Autodesk Inventor part; units mm, degrees
ref_plane "YZ Plane" through (0, 0, 0) normal (1, 0, 0) x (0, 1, 0)
ref_plane "XZ Plane" through (0, 0, 0) normal (0, 1, 0) x (-1, 0, 0)
ref_plane "XY Plane" through (0, 0, 0) normal (0, 0, 1) x (1, 0, 0)
sketch "Sketch2" plane through (0, 0, 0) normal (0, 1, 0) x (-1, 0, 0)
  line L0 (0, 0) -> (100, 0)
  line L1 (100, 0) -> (100, -100)
  line L2 (100, -100) -> (0, -100)
  line L3 (0, -100) -> (0, 0)
  dimension "d2" = 100
  dimension "d3" = 100
extrude "Extrusion2" add sketch "Sketch2" along normal blind 3
sketch "Sketch3" plane through (0, 0, 0) normal (1, 0, 0) x (0, 0, -1)
  line L0 (0, 0) -> (100, 0)
  line L1 (100, 0) -> (100, 113)
  line L2 (100, 113) -> (0, 113)
  line L3 (0, 113) -> (0, 0)
  dimension "d6" = 100
  dimension "d7" = 113
extrude "Extrusion3" add sketch "Sketch3" along normal blind 3
sketch "Sketch4" plane through (0, 3, 0) normal (0, 0, 1) x (1, 0, 0)
  line L0 (3, -3) -> (-100, -3)
  line L1 (3, -3) -> (-100, -3)
  line L2 (-100, -3) -> (-100, 110)
  line L3 (-100, 110) -> (3, 110)
  line L4 (3, 110) -> (3, -3)
  point P0 (0, -3)
  dimension "d10" = 113
  dimension "d11" = 103
extrude "Extrusion4" add sketch "Sketch4" along normal blind 3
sketch "Sketch5" plane through (-100, 3, 0) normal (-1, 0, 0) x (0, 0, 1)
  line L0 (-100, -3) -> (3, -3)
  line L1 (-100, 110) -> (3, 110)
  line L2 (3, -3) -> (-100, -3)
  line L3 (-100, -3) -> (-100, 110)
  line L4 (-100, 110) -> (3, 110)
  line L5 (3, 110) -> (3, -3)
  point P0 (0, -3)
  point P1 (3, 110)
extrude "Extrusion5" add sketch "Sketch5" along normal blind 3
sketch "Sketch6" plane through (0, 3, -100) normal (0, 0, -1) x (-1, 0, 0)
  line L0 (103, -3) -> (103, 110)
  line L1 (-3, -3) -> (103, -3)
  line L2 (103, -3) -> (103, 97)
  line L3 (103, 97) -> (-3, 97)
  line L4 (-3, 97) -> (-3, -3)
  point P0 (0, -3)
  dimension "d16" = 100
extrude "Extrusion6" add sketch "Sketch6" along normal blind 3
sketch "Sketch7" plane through (3, 0, 0) normal (1, 0, 0) x (0, 0, -1)
  point P0 (0, 0)
ref_plane "Work Plane1" through (-50, 3, 0) normal (1, 0, 0) x (0, 0, -1)
sketch "Sketch8" plane through (-50, 3, 0) normal (1, 0, 0) x (0, 0, -1)
  line L0 (103, 97) -> (103, -3)
  line L1 (103, 97) -> (133.6418, 71.2885)
  line L2 (133.6418, 71.2885) -> (133.6418, 31.2885)
  line L3 (130.6418, 69.8896) -> (103, 93.0838)
  line L4 (133.6418, 31.2885) -> (130.6418, 51.2885)
  line L5 (130.6418, 51.2885) -> (130.6418, 69.8896)
  line L6 (103, 93.0838) -> (100, 95.6011)
  line L7 (100, 0) -> (100, 97)
  line L8 (100, 97) -> (103, 97)
  line L9 (103, 97) -> (103, 110)
  line L10 (100, 110) -> (100, 97)
  line L11 (103, 110) -> (100, 110)
  line L12 (100, 110) -> (100, 95.6011)
  line L13 (100, 95.6011) -> (100, 97)
  line L14 (140.6418, 31.2885) -> (140.6418, 72.7039) construction
  point P0 (0, -3)
  dimension "d20" = 40
  dimension "d21" = 50
  dimension "d22" = 40
  dimension "d24" = 3
  dimension "d27" = 20
  dimension "d28" = 18.6011
  dimension "d29" = 7
revolve "Revolution1" add sketch "Sketch8" angle 360 about axis through (-50, 34.2885, -140.6418) along (0, 1, 0)
ref_plane "Work Plane2" through (-50, 63.589, -130.6418) normal (0, 0, -1) x (-1, 0, 0)
sketch "Sketch9" plane through (-50, 63.589, -130.6418) normal (0, 0, -1) x (-1, 0, 0)
  line L0 (-15.3248, 36.411) -> (-53, 36.411)
  line L1 (-50, 49.411) -> (50, 49.411)
  line L2 (-40.4865, 36.411) -> (40.6129, 36.411)
  line L3 (40.6129, 36.411) -> (40.6129, 49.411)
  line L4 (40.6129, 49.411) -> (-40.4865, 49.411)
  line L5 (-40.4865, 49.411) -> (-40.4865, 36.411)
  point P0 (-50, -63.589)
extrude "Extrusion7" cut sketch "Sketch9" against normal up to surface (130.6418 mm away)
sketch "Sketch10" plane through (-100, 100, -100) normal (0, 1, 0) x (1, 0, 0)
  line L0 (89.3923, 30.6418) -> (86.2892, 30.6418)
  line L1 (103, 0) -> (103, 3)
  line L2 (89.3923, 30.6418) -> (103, 3)
  line L3 (-3, 3) -> (34.6752, 3)
  line L4 (103, 3) -> (-3, 3)
  line L5 (-3, 3) -> (10.6077, 30.6418)
  arc A0 (65.3248, 3) -> (34.6752, 3) centre (50, 40.6418) ccw
  point P0 (100, -100)
extrude "Extrusion8" add sketch "Sketch10" against normal blind 1.5 contours L2 L4 A0 | A0 L3 L5
sketch "Sketch11" plane through (-103, 100, -100) normal (0, 1, 0) x (1, 0, 0)
  line L0 (92.3923, 30.6418) -> (89.2892, 30.6418)
  line L1 (103, 0) -> (89.2892, 30.6418)
  arc A0 (68.3248, 3) -> (92.3923, 30.6418) centre (53, 40.6418) ccw
  line L2 (89.2892, 30.6418) -> (92.3923, 30.6418)
  line L3 (106, 3) -> (92.3923, 30.6418)
  line L4 (92.3923, 30.6418) -> (106, 3)
  line L5 (106, 0) -> (103, 0)
  line L6 (106, 3) -> (106, 0)
  line L7 (106, 0) -> (103, 0)
  line L8 (16.7108, 30.6418) -> (13.6077, 30.6418)
  line L9 (3, -100) -> (3, 0)
  line L10 (16.7108, 30.6418) -> (3, 0)
  line L11 (3, 0) -> (0, 0)
  line L12 (0, 0) -> (0, 3)
  line L13 (0, 0) -> (0, 3)
  line L14 (13.6077, 30.6418) -> (16.7108, 30.6418)
  line L15 (16.7108, 30.6418) -> (13.6077, 30.6418)
  line L16 (13.6077, 30.6418) -> (0, 3)
  point P0 (103, -100)
  dimension "d35" = 30.8097
extrude "Extrusion9" add sketch "Sketch11" along normal blind 13
ref_plane "Work Plane3" through (0, 3, -13) normal (0, 0, -1) x (-1, 0, 0)
sketch "Sketch13" plane through (-50, 3, 0) normal (1, 0, 0) x (0, 0, -1)
  line L0 (100, 0) -> (0, 0)
  line L1 (24, 0) -> (-2.4904, 18.5488)
  line L2 (-2.4904, 18.5488) -> (-0.7697, 21.0062)
  line L3 (-0.7697, 21.0062) -> (29.2303, 0)
  line L4 (12.4755, 11.7318) -> (125.6722, 173.3935)
  point P0 (0, -3)
  dimension "d39" = 35
  dimension "d41" = 3
  dimension "d42" = 30
  dimension "d44" = 24
  dimension "d54" = 90
extrude "Extrusion10" add sketch "Sketch13" along normal mid plane 30
sketch "Sketch21" plane through (-50, 3, 0) normal (1, 0, 0) x (0, 0, -1)
  line L0 (100, 97) -> (73.837, 123.163)
  line L1 (100, 97) -> (100, 0)
  line L2 (73.837, 123.163) -> (71.7157, 121.0416)
  line L3 (71.7157, 121.0416) -> (100, 92.7574)
  point P0 (0, -3)
  dimension "d55" = 45
  dimension "d56" = 3
  dimension "d57" = 40
  dimension "d59" = 90
extrude "Extrusion12" add sketch "Sketch21" along normal mid plane 30
ref_plane "Work Plane4" through (-65, 21.0098, 1.7207) normal (0, 0.8192, -0.5736) x (1, 0, 0)
sketch "Sketch24" plane through (-65, 21.0098, 1.7207) normal (0, 0.8192, -0.5736) x (1, 0, 0)
  line L0 (0, 35.6837) -> (30, 35.6837) construction
  line L1 (15, 35.6837) -> (15, 2.1006) construction
  line L2 (0, 2.1006) -> (30, 2.1006) construction
  circle A0 centre (15, 18.8921) radius 11
  point P0 (65, 13.4603)
  dimension "d63" = 22
extrude "Extrusion13" cut sketch "Sketch24" along normal through all
sketch "Sketch25" plane through (-65, 3, 0) normal (-1, 0, 0) x (0, 0, 1)
  line L0 (-71.7157, 121.0416) -> (-73.837, 123.163)
  line L1 (-71.7157, 121.0416) -> (-100.9447, 80.4748)
  line L2 (-100, 92.7574) -> (-71.7157, 121.0416)
  line L3 (-100.9447, 80.4748) -> (-100, 97)
  line L4 (-73.837, 123.163) -> (-100, 97)
  line L5 (-73.837, 123.163) -> (-71.7157, 121.0416)
  point P0 (0, -3)
  dimension "d66" = 50
  dimension "d67" = 170.773
extrude "Extrusion14" add sketch "Sketch25" against normal blind 3
sketch "Sketch26" plane through (-35, 3, 0) normal (1, 0, 0) x (0, 0, -1)
  line L0 (71.7157, 121.0416) -> (100, 92.7574)
  line L1 (100, 81.786) -> (71.7157, 121.0416)
  line L2 (71.7157, 121.0416) -> (100, 81.786)
  line L3 (100, 81.786) -> (100, 92.7574)
  line L4 (71.7157, 121.0416) -> (73.837, 123.163)
  line L5 (100, 92.7574) -> (71.7157, 121.0416)
  point P0 (0, -3)
extrude "Extrusion15" add sketch "Sketch26" against normal blind 3
equation "\"d3\" = d2"
equation "\"d16\" = d2"
properties part number "resoar"
Check sheet for the modelled part. Datum: model origin and axes. Units: mm. A direction names the side the tool comes from. Round coordinates to 2 decimals unless told otherwise and drop trailing zeros. Loops run counter-clockwise (first coordinate to the right, second up) from the corner with the lowest first, then second, coordinate; pieces in that order, holes last. Notation, with made-up numbers: (34, 33) - (40, 33) arc R23 ccw to (40, 69) - close; hole circle Ø5 at (74.25, 74). An arc over 180 degrees is marked (long way). Answer as CSV lines item,"result". Start each with the question number.
Item 1: Release check for a two-part mould opening along Y. For faces 4 (the flat face through (-36.479, 104.139, -86.056)), 5 (the flat face through (-49, 50, -103)), 6 (the flat face through (-56.88, 17.93, -7.91)), 7 (the flat face through (-55.5, 103.81, -91.95)) record: +Y half, -Y half, draft (parallel to the pull), parting line (faces both ways), or undercut.
Item 2: Section check C-C (y = 81). Record the boundary of the cut face in (x, z), and give its area (3 significant figures).
Item 3: Depth check by flat-ended pin: P1, Ø10, axis at x = -81, z = -92, coming from the -Y side; P2, Ø22, axis at x = -7, z = -123, coming from the -Y side; P3, Ø5, axis at x = -71, y = 42.5, coming from the -Z side; P4, Ø8.5, axis at x = -50, z = -140.64, coming from the -Y side. Enter the tip coordinate at first touch or a pass-through.
Item 4: Scan lines: line 1 (X direction, y = 36.5, z = -80); line 2 (Z direction, x = -65.5, y = 96.5). Record each from-to range of solid material in increasing order. Write a range as [from, to].
Item 5: Section check A-A (y = 66.5). Record the boundary of the cut face in (x, z).
Item 6: Section check B-B (z = -41). Record the boundary of the cut face in (x, y), and give its area (3 significant figures).
Item 7: Set-up check for faces 1 (the flat face through (-62, 102, -89)), 2 (the flat face through (-6.76, 106.41, -115.11)), 3 (the cylindrical face through (-53.83, 63.719, -131.404)): record each of +Z, -Z, +X, -X, +Y, -Y from which the full face is reachable in a straight line by a thin tool's end or side.
Item 8: Section check D-D (x = -3). Record the boundary of the cut face in (y, z), and give its area (3 significant figures).
Report:
1,face 4,"undercut"
1,face 5,"draft"
1,face 6,"+Y half"
1,face 7,"undercut"
2,outline,"(-103, -103) - (3, -103) - (3, 3) - (-103, 3) - close; circle Ø39.33 at (-50, -140.64); hole (-100, -100) - (0, -100) - (0, 0) - (-100, 0) - close; hole circle Ø30 at (-50, -140.64)"
2,area,"1,740 mm2"
3,P1,"stops at y = 0"
3,P2,"stops at y = 94.27"
3,P3,"stops at z = -103"
3,P4,"passes through"
4,line 1,"x = [-103, -100], [0, 3]"
4,line 2,"z = [-175.49, -170.31], [-110.98, -105.8], [-103, -100], [0, 3]"
5,outline,"(-103, -103) - (3, -103) - (3, 3) - (-103, 3) - close; circle Ø20 at (-50, -140.64); hole (-100, -100) - (0, -100) - (0, 0) - (-100, 0) - close; hole circle Ø14 at (-50, -140.64)"
6,outline,"(-103, 0) - (3, 0) - (3, 113) - (0, 113) - (0, 3) - (-100, 3) - (-100, 113) - (-103, 113) - close"
6,area,"978 mm2"
7,face 1,"none"
7,face 2,"+Y"
7,face 3,"-Y"
8,outline,"(0, -103) - (98.5, -103) - (98.5, -115.19) - (113, -115.19) - (113, -106.7) - (100, -106.7) - (100, -100) - (3, -100) - (3, 0) - (113, 0) - (113, 3) - (0, 3) - close"
8,area,"1,070 mm2"
